Build history of the part. All positions in model axes, mm. A direction names the side the tool comes from. Give positions to 0.01 mm unless a question says otherwise; leave off trailing zeros. Order: outer loops, then holes, each group sorted by start corner. A loop starts at its lowest first (then second) coordinate and runs counter-clockwise, first axis right, second up. Notation, with made-up numbers: (57, 31) - (85, 31) arc R23 cw to (85, 49) - close; hole circle Ø2 at (82, 71). An arc over 180 degrees is marked (long way). Answer in a Markdown table with one row per item.
```python
from build123d import *

# Parameters (mm, degrees)
F0_W     = 32
F0_H     = 24
F1_DEPTH = 32
F2_W     = 8
F2_H     = 8
F3_DEPTH = 24
F4_W     = 32
F4_H     = 32
F5_DEPTH = 8


with BuildPart() as f1:
    # F0 (on Front) → F1 (new body)
    with BuildSketch(Plane.XZ):
        Rectangle(F0_W, F0_H)
    extrude(amount=F1_DEPTH)

    # F2 (on face) → F3 (join)
    with BuildSketch(Plane.XY.offset(12)):
        with Locations((0, -16)):
            Rectangle(F2_W, F2_H)
    extrude(amount=F3_DEPTH)

    # F4 (on face) → F5 (join)
    with BuildSketch(Plane.XY.offset(36)):
        with Locations((-0.237114, -16)):
            Rectangle(F4_W, F4_H)
    extrude(amount=F5_DEPTH)


solid = f1.part
```
1. Drop flat-ended pins along their axis: P1, Ø2.5, axis at y = -13, z = 41, coming from the +X side; P2, Ø7, axis at y = -12, z = -3.5, coming from the -X side; P3, Ø9, axis at x = -0.5, z = 22, coming from the -Y side. Give the stop position or say it passes through.
Check result:
| item | result |
|---|---|
| P1 | stops at x = 15.76 |
| P2 | stops at x = -16 |
| P3 | stops at y = -20 |
2. Two-plate mould, pull along Z, no slides. Class faces 1 (the face through (0, -12, 24)), 2 (the face through (0, -16, 44)), 3 (the face through (0, 0, 0)): +Z half, -Z half, draft (parallel to the pull), parting line (faces both ways), or undercut.
Check result:
| item | result |
|---|---|
| face 1 | undercut |
| face 2 | +Z half |
| face 3 | draft |
3. Cut at A-A on x = 7.5. Write the cut outline in (y, z), and give its area (3 significant figures).
Check result:
| item | result |
|---|---|
| outline | (-32, -12) - (0, -12) - (0, 12) - (-32, 12) - close; (-32, 36) - (0, 36) - (0, 44) - (-32, 44) - close |
| area | 1,020 mm² |
4. Probe line 1 (Z direction, x = 2, y = -3); line 2 (Y direction, x = 3, z = 13); line 3 (X direction, y = -17, z = 30). List the from-to ranges inside material, lowest first.
Check result:
| item | result |
|---|---|
| line 1 | z = -12 to 12, 36 to 44 |
| line 2 | y = -20 to -12 |
| line 3 | x = -4 to 4 |
5. Cut at D-D on x = 1. Write the cut outline in (y, z), and give its area (3 significant figures).
Check result:
| item | result |
|---|---|
| outline | (-32, -12) - (0, -12) - (0, 12) - (-12, 12) - (-12, 36) - (0, 36) - (0, 44) - (-32, 44) - (-32, 36) - (-20, 36) - (-20, 12) - (-32, 12) - close |
| area | 1,220 mm² |
6. Cut at B-B on y = -6. Write the cut outline in (x, z), and give its area (3 significant figures).
Check result:
| item | result |
|---|---|
| outline | (-16.24, 36) - (15.76, 36) - (15.76, 44) - (-16.24, 44) - close; (-16, -12) - (16, -12) - (16, 12) - (-16, 12) - close |
| area | 1,020 mm² |
7. Cut at C-C on y = -17. Write the cut outline in (x, z).
Check result:
| item | result |
|---|---|
| outline | (-16.24, 36) - (-4, 36) - (-4, 12) - (-16, 12) - (-16, -12) - (16, -12) - (16, 12) - (4, 12) - (4, 36) - (15.76, 36) - (15.76, 44) - (-16.24, 44) - close |
8. Which spindle directions (+Z, -Z, +X, -X, +Y, -Y) get a long thin tool onto all of the face, cutting with end or side? Do faces 4 (the face through (-16, -16, 0)), 5 (the face through (4, -16, 24)), 6 (the face through (0, -23, 12)), 7 (the face through (15.763, -16, 40)). Say none if no direction does.
Check result:
| item | result |
|---|---|
| face 4 | -Z, -X, +Y, -Y |
| face 5 | +X, +Y, -Y |
| face 6 | none |
| face 7 | +Z, +X, +Y, -Y |
